The figure shows three views and two pictorial views of one solid part (mm, origin at its lowest corner). Answer the questions. A direction names the side the tool comes from. Coordinates: 2 decimals unless noted, no trailing zeros. Order: outer loops, then holes, each group sorted by start corner. A loop starts at its lowest first (then second) coordinate and runs counter-clockwise, first axis right, second up. Notation, with made-up numbers: (23, -37) - (41, -37) arc R19 ccw to (41, -19) - close; hole circle Ø10 at (-36, -14.75). An arc over 180 degrees is marked (long way). Use one line per item in the form item = value. Start each with the question number.
Item 1: Consider line 1 along X through (y, z) = (194, 36). Determine where the line is inside the solid, lowest interval first. Write a range as [from, to].
Item 2: Section A-A, the plane z = 70.5 is taken. Write down the section's boundary in (x, y), and give its area (3 significant figures).
Item 3: This flat-tipped pin is pushed along its axis until it touches: pin 1 Ø4 at (y, z) = (201.5, 23) entering from +X. Where does it stop, or does it pass through?
Item 4: A tool of negligible diameter and unlimited length cuts with its end or side. For the marked faces 1 and 2, from which of +Z, -Z, +X, -X, +Y, -Y can it reach the whole face along a straight path? Write none if from no direction.
Item 5: Section B-B, the plane x = 167 is taken. Write down the section's boundary in (y, z), and give its area (3 significant figures).
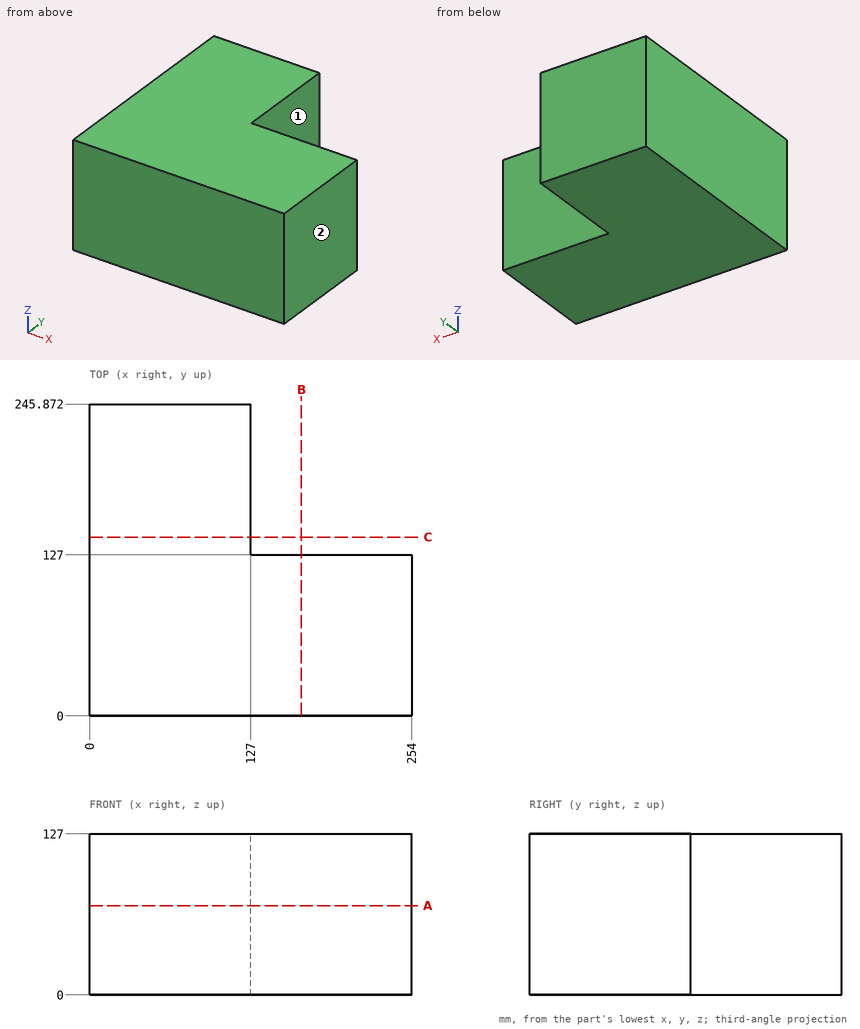
Response:
q1.line_1 = [0, 127]
q2.outline = (0, 0) - (254, 0) - (254, 127) - (127, 127) - (127, 245.87) - (0, 245.87) - close
q2.area = 47,400 mm2
q3.pin_1 = 127
q4.face_1 = +Z, -Z, +X, +Y
q4.face_2 = +Z, -Z, +X, +Y, -Y
q5.outline = (0, 0) - (127, 0) - (127, 127) - (0, 127) - close
q5.area = 16,100 mm2
